Read the model definition and answer for the solid it produces. Units are mm, in the model's axes. A direction names the side the tool comes from. Round coordinates to 2 decimals unless told otherwise and drop trailing zeros. Write each loop counter-clockwise with the first axis right and the second up, starting at its lowest first coordinate (ties: lowest second). Pieces come first, ordered by that corner, then holes.
from build123d import *

# Parameters (mm, degrees)
SKETCH_1_W               = 40
SKETCH_1_H               = 30
SKETCH_1_W_2             = 38
SKETCH_1_H_2             = 28
EXTRUDE_1_DEPTH          = 95
CUT_EXTRUDE_1_DEPTH      = 102.612007165
CUT_EXTRUDE_1_DEPTH_BACK = 102.612007165
SKETCH_2_R               = 1.6
SKETCH_3_R               = 1.6
CUT_EXTRUDE_2_DEPTH      = 105.16333328


with BuildPart() as part:
    # 草图1 → 凸台-拉伸1 (new, symmetric)
    with BuildSketch(Plane(origin=(0, 0, 0), x_dir=(0, 0, -1), z_dir=(1, 0, 0))):
        Rectangle(SKETCH_1_W, SKETCH_1_H)
        Rectangle(SKETCH_1_W_2, SKETCH_1_H_2, mode=Mode.SUBTRACT)
    extrude(amount=EXTRUDE_1_DEPTH, both=True)

    # 草图2 → 切除-拉伸1 (cut, two sides: drawn at the far end of the back side and taken through both)
    with BuildSketch(Plane(origin=(0, 15, 0), x_dir=(1, 0, 0), z_dir=(0, 1, 0)).offset(-CUT_EXTRUDE_1_DEPTH_BACK)):
        with Locations(Location((0, -13, 0), (0, 0, 270))):
            Circle(SKETCH_2_R)
        with Locations(Location((-33, 10, 0), (0, 0, 270))):
            Circle(SKETCH_2_R)
        with Locations(Location((33, 10, 0), (0, 0, 270))):
            Circle(SKETCH_2_R)
        with Locations(Location((-85, 15, 0), (0, 0, 270))):
            Circle(SKETCH_2_R)
        with Locations(Location((-85, -15, 0), (0, 0, 270))):
            Circle(SKETCH_2_R)
        with Locations(Location((85, -15, 0), (0, 0, 270))):
            Circle(SKETCH_2_R)
        with Locations(Location((85, 15, 0), (0, 0, 270))):
            Circle(SKETCH_2_R)
    extrude(amount=CUT_EXTRUDE_1_DEPTH + CUT_EXTRUDE_1_DEPTH_BACK, mode=Mode.SUBTRACT)

    # 草图3 → 切除-拉伸2 (cut, through all)
    with BuildSketch(Plane.XY.offset(20)):
        with Locations((-90, 10)):
            Circle(SKETCH_3_R)
        with Locations(Location((-90, -10, 0), (0, 0, 270))):
            Circle(SKETCH_3_R)
        with Locations((-80, 10)):
            Circle(SKETCH_3_R)
        with Locations(Location((-80, -10, 0), (0, 0, 270))):
            Circle(SKETCH_3_R)
        with Locations((80, -10)):
            Circle(SKETCH_3_R)
        with Locations(Location((80, 10, 0), (0, 0, 270))):
            Circle(SKETCH_3_R)
        with Locations((90, -10)):
            Circle(SKETCH_3_R)
        with Locations(Location((90, 10, 0), (0, 0, 270))):
            Circle(SKETCH_3_R)
    extrude(amount=-CUT_EXTRUDE_2_DEPTH, mode=Mode.SUBTRACT)


solid = part.part
Q1. Section B-B (y = -2.25) is taken. Determine the outline of the cut face in (x, z).
Verdict:
outline: (-95, -20) - (95, -20) - (95, -19) - (-95, -19) - close; (-95, 19) - (95, 19) - (95, 20) - (-95, 20) - close
Q2. Section D-D (z = 8.5) is taken. Determine the outline of the cut face in (x, y).
Verdict:
outline: (-95, -15) - (95, -15) - (95, -14) - (-95, -14) - close; (-95, 14) - (95, 14) - (95, 15) - (-95, 15) - close
Q3. Section A-A (x = 33) is taken. Determine the outline of the cut face in (y, z), then the cut area to 3 significant figures.
Verdict:
outline: (-15, -20) - (15, -20) - (15, -11.6) - (14, -11.6) - (14, -19) - (-14, -19) - (-14, -11.6) - (-15, -11.6) - close; (-15, -8.4) - (-14, -8.4) - (-14, 19) - (14, 19) - (14, -8.4) - (15, -8.4) - (15, 20) - (-15, 20) - close
area: 130 mm2
Q4. Determine the mould class of faces 1 (the flat face through (1, 0, -20)), 2 (the cylindrical face through (-34.56, 14.49, -10.35)), 3 (the flat face through (1, 15, 0)) for opening direction Z: pulls with the +Z half, pulls with the -Z half, needs draft (parallel to the pull), parting line crosses it, or undercut.
Verdict:
face 1: pulls with the -Z half
face 2: undercut
face 3: needs draft
Q5. Section C-C (x = -80) is taken. Determine the outline of the cut face in (y, z), then the cut area to 3 significant figures.
Verdict:
outline: (-15, -20) - (-11.6, -20) - (-11.6, -19) - (-14, -19) - (-14, 19) - (-11.6, 19) - (-11.6, 20) - (-15, 20) - close; (-8.4, -20) - (8.4, -20) - (8.4, -19) - (-8.4, -19) - close; (-8.4, 19) - (8.4, 19) - (8.4, 20) - (-8.4, 20) - close; (11.6, -20) - (15, -20) - (15, 20) - (11.6, 20) - (11.6, 19) - (14, 19) - (14, -19) - (11.6, -19) - close
area: 123 mm2
Q6. Flat-ended cylindrical pins translate along their axes: pin 1 Ø4 at (x, z) = (0, 13) entering from -Y; pin 2 Ø1.9 at (x, z) = (33, -10) entering from -Y. Find the tip coordinate at first contact, or state that the pin passes through.
Verdict:
pin 1: stops at y = -15
pin 2: passes through
Q7. Straight lines are drawn through the part: probe 1 along Y at (x, z) = (90, 19.3); probe 2 along Y at (x, z) = (-42, -6.5); probe 3 along Z at (x, y) = (85, 14.5). For each, find the intervals that lie inside material, in ascending order.
Verdict:
probe 1: y = -15 to -11.6, -8.4 to 8.4, 11.6 to 15
probe 2: y = -15 to -14, 14 to 15
probe 3: z = -20 to -16.6, -13.4 to 13.4, 16.6 to 20
Q8. Which of the six approach directions +Z, -Z, +X, -X, +Y, -Y give full straight-line access (tool end or side, diameter ignored) to faces 4 (the cylindrical face through (-84.93, 14.49, 13.4)), 5 (the flat face through (1, 0, 19))?
Verdict:
face 4: +Y, -Y
face 5: +X, -X
